Geometry check sheet. Reference: the model listing, model coordinates, mm. Face numbers are marked on the shaded views. A direction names the side the tool comes from. Give positions to 0.01 mm unless a question says otherwise; leave off trailing zeros. Write each loop counter-clockwise with the first axis right and the second up, starting at its lowest first coordinate (ties: lowest second). Pieces come first, ordered by that corner, then holes. Notation, with made-up numbers: M 4.5,58 L 48.5,58 A7 cw 48.5,64 Z; hole C 41,85 d8. An arc over 180 degrees is marked long. One line per item, written item: value. Start each with the question number.
1. Cross-section at C-C on x = 0.25. Record the cut outline in (y, z).
2. Cross-section at B-B on z = 0.4. Record the cut outline in (x, y), then the cut area to 3 significant figures.
3. Gauge pin test, flat ends, axial feed: pin 1 (1.5 mm diameter, centred on x = -2, y = 9.5, fed in from +Z); pin 2 (2.5 mm diameter, centred on x = 1.04, y = -8, fed in from +Z) (3 decimals); pin 3 (3.5 mm diameter, centred on x = 1.04, y = 8, fed in from -Z); pin 4 (1.2 mm diameter, centred on x = -6.5, z = 1, fed in from -Y). Record the tip position at first contact, or that the pin passes through.
4. Scan lines: line 1 (Z direction, x = -3.25, y = 9.25); line 2 (Y direction, x = -7, z = -0.75); line 3 (X direction, y = 5, z = 1.5). Record each from-to range of solid material in increasing order.
5. Cross-section at D-D on z = 1.6. Record the cut outline in (x, y).
6. Tool access check on the marked faces 1, 2, 3 and 4. Record the directions out of +Z, -Z, +X, -X, +Y, -Y that give a thin tool (end or side, any length) a straight path to the whole face; none if there is none.
7. Cross-section at A-A on y = -8. Record the cut outline in (x, z).
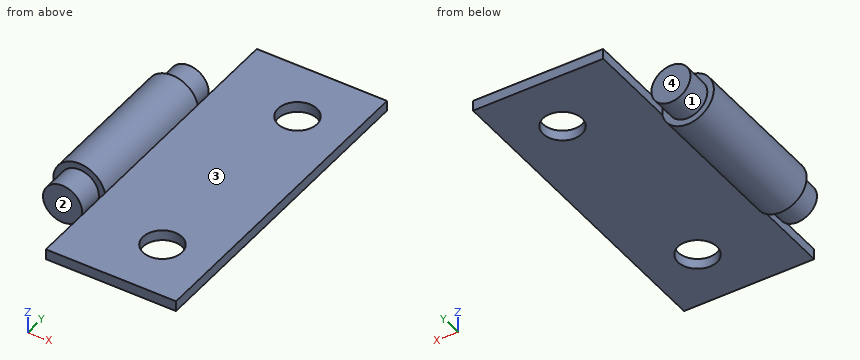
from build123d import *

# Parameters (mm, degrees)
SKETCH_1_W          = 10
SKETCH_1_H          = 25
EXTRUDE_1_DEPTH     = 0.8
SKETCH_4_R          = 2
EXTRUDE_2_DEPTH     = 5.5
SKETCH_5_R          = 1.5
EXTRUDE_3_DEPTH     = 2
SKETCH_6_R          = 1.5
CUT_EXTRUDE_1_DEPTH = 4


with BuildPart() as part:
    # 草图1 → 凸台-拉伸1 (new body)
    with BuildSketch(Plane.XY):
        Rectangle(SKETCH_1_W, SKETCH_1_H)
    extrude(amount=EXTRUDE_1_DEPTH)

    # 草图4 → 凸台-拉伸2 (add, symmetric)
    with BuildSketch(Plane(origin=(0, 0, 0), x_dir=(1, 0, 0), z_dir=(0, 1, 0))):
        with Locations((-6.959591794, -0.4)):
            Circle(SKETCH_4_R)
    extrude(amount=EXTRUDE_2_DEPTH, both=True)

    # 草图5 → 凸台-拉伸3 (add, symmetric)
    with BuildSketch(Plane(origin=(0, 5.5, 0), x_dir=(1, 0, 0), z_dir=(0, 1, 0))):
        with Locations(Location((-6.959591794, -0.4, 0), (0, 0, 270))):
            Circle(SKETCH_5_R)
    extrude_3 = extrude(amount=EXTRUDE_3_DEPTH, both=True)

    # 镜向1: 凸台-拉伸3 across plane
    add(extrude_3.mirror(Plane.ZX))

    # 草图6 → 切除-拉伸1 (cut)
    with BuildSketch(Plane(origin=(0, 0, 0), x_dir=(-1, 0, 0), z_dir=(0, 0, -1))):
        with Locations((-1.040408206, 8)):
            Circle(SKETCH_6_R)
        with Locations((-1.040408206, -8)):
            Circle(SKETCH_6_R)
    extrude(amount=-CUT_EXTRUDE_1_DEPTH, mode=Mode.SUBTRACT)


solid = part.part
Report:
1. outline: M -12.5,0 L -9.27,0 L -9.27,0.8 L -12.5,0.8 Z; M -6.73,0 L 6.73,0 L 6.73,0.8 L -6.73,0.8 Z; M 9.27,0 L 12.5,0 L 12.5,0.8 L 9.27,0.8 Z
2. outline: M -8.96,-5.5 L -8.46,-5.5 L -8.46,-7.5 L -5.46,-7.5 L -5.46,-5.5 L -5,-5.5 L -5,-12.5 L 5,-12.5 L 5,12.5 L -5,12.5 L -5,5.5 L -5.46,5.5 L -5.46,7.5 L -8.46,7.5 L -8.46,5.5 L -8.96,5.5 Z; hole C 1.04,-8 d3; hole C 1.04,8 d3
2. area: 291 mm^2
3. pin 1: stops at z = 0.8
3. pin 2: passes through
3. pin 3: stops at z = 0
3. pin 4: stops at y = -7.5
4. line 1: z = 0 to 0.8
4. line 2: y = -7.5 to 7.5
4. line 3: x = -8.63 to -5.29
5. outline: M -8.56,-5.5 L -7.86,-5.5 L -7.86,-7.5 L -6.06,-7.5 L -6.06,-5.5 L -5.36,-5.5 L -5.36,5.5 L -6.06,5.5 L -6.06,7.5 L -7.86,7.5 L -7.86,5.5 L -8.56,5.5 Z
6. face 1: +Y
6. face 2: +Z, -Z, -X, -Y
6. face 3: +Z, +X, +Y, -Y
6. face 4: +Z, -Z, -X, +Y
7. outline: M -5,0 L -0.46,0 L -0.46,0.8 L -5,0.8 Z; M 2.54,0 L 5,0 L 5,0.8 L 2.54,0.8 Z
